Input: part model. Units: mm. Frame: model coordinates. Give positions to 0.01 mm unless a question says otherwise; leave off trailing zeros. Write each loop counter-clockwise with the first axis right and the second up, starting at its lowest first coordinate (ties: lowest second). Pieces come first, ordered by that corner, then holes. Notation, with made-up numbers: (-22, 32.25) - (21, 32.25) arc R23 cw to (21, 53.25) - close; hole circle Ø11 at (77.25, 60). An arc over 180 degrees is marked (long way). Answer as CSV lines item,"result".
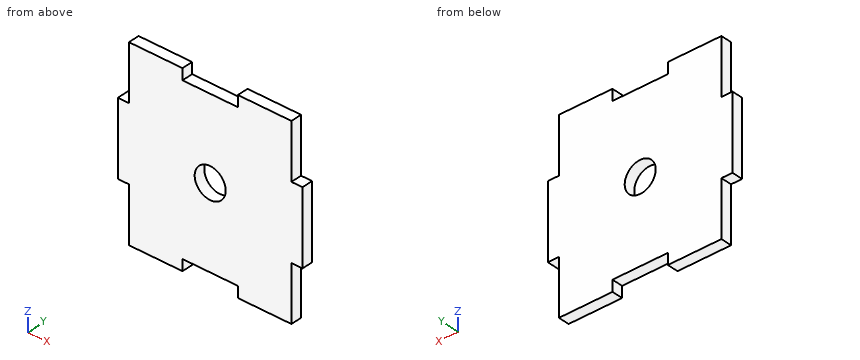
```python
from build123d import *

# Parameters (mm, degrees)
SKETCH_1_R      = 4.2
EXTRUDE_1_DEPTH = 3


with BuildPart() as part:
    # 草图1 → 凸台-拉伸1 (new body)
    with BuildSketch(Plane(origin=(0, 0, 0), x_dir=(1, 0, 0), z_dir=(0, 1, 0))):
        Polygon((22, 25), (22, 10), (25, 10), (25, -10), (22, -10), (22, -25), (7.5, -25), (7.5, -22), (-7.5, -22), (-7.5, -25), (-22, -25), (-22, -10), (-25, -10), (-25, 10), (-22, 10), (-22, 25), (-7.5, 25), (-7.5, 22), (7.5, 22), (7.5, 25), align=None)
        Circle(SKETCH_1_R, mode=Mode.SUBTRACT)
    extrude(amount=EXTRUDE_1_DEPTH)


solid = part.part
```
Item 1: Cut plane D-D on z = 19. Return the cut outline in (x, y), plus the area to 3 significant figures.
The answers:
outline,"(-22, 0) - (22, 0) - (22, 3) - (-22, 3) - close"
area,"132 mm²"
Item 2: Contact query for flat-ended pins moving along their axis: pin 1 (1.5 mm diameter, centred on x = -1.5, y = 1.5, fed in from -Z); pin 2 (1.5 mm diameter, centred on y = 1.5, z = -24, fed in from -X); pin 3 (0.9 mm diameter, centred on x = 24, y = 2, fed in from -Z). Output: stop coordinate, or through.
The answers:
pin 1,"z = -22"
pin 2,"x = -22"
pin 3,"z = -10"
Item 3: Ray query, line 1 (X direction, y = 1.55, z = 0); line 2 (Z direction, x = 0, y = 2.15); line 3 (X direction, y = 0.5, z = -16.5). Return the intervals inside material, ascending. Write a range as from..to.
The answers:
line 1,"-25..-4.2, 4.2..25"
line 2,"-22..-4.2, 4.2..22"
line 3,"-22..22"
Item 4: Cut plane A-A on x = 0. Return the cut outline in (y, z), plus the area to 3 significant figures.
The answers:
outline,"(0, -22) - (3, -22) - (3, -4.2) - (0, -4.2) - close; (0, 4.2) - (3, 4.2) - (3, 22) - (0, 22) - close"
area,"107 mm²"
Item 5: Cut plane C-C on y = 0.8. Return the cut outline in (x, z).
The answers:
outline,"(-25, -10) - (-22, -10) - (-22, -25) - (-7.5, -25) - (-7.5, -22) - (7.5, -22) - (7.5, -25) - (22, -25) - (22, -10) - (25, -10) - (25, 10) - (22, 10) - (22, 25) - (7.5, 25) - (7.5, 22) - (-7.5, 22) - (-7.5, 25) - (-22, 25) - (-22, 10) - (-25, 10) - close; hole circle Ø8.4 at (0, 0)"
Item 6: Cut plane B-B on z = 0. Return the cut outline in (x, y), plus the area to 3 significant figures.
The answers:
outline,"(-25, 0) - (-4.2, 0) - (-4.2, 3) - (-25, 3) - close; (4.2, 0) - (25, 0) - (25, 3) - (4.2, 3) - close"
area,"125 mm²"
